from build123d import *

# Parameters (mm, degrees)
PAD004_DEPTH = 0.25
PAD003_DEPTH = 0.25
PAD005_DEPTH = 0.25
PAD008_DEPTH = 0.3
SKETCH008_W  = 4.5
SKETCH008_H  = 0.35
PAD006_DEPTH = 4
PAD001_DEPTH = 0.18
PAD002_DEPTH = 0.25
PAD007_DEPTH = 0.3
SKETCH_W     = 10
SKETCH_H     = 6.5
PAD_DEPTH    = 4.7
POCKET_DEPTH = 0.5
FILLET_R     = 0.2


with BuildPart() as pad004:
    # Sketch006 → Pad004 (new body, symmetric)
    with BuildSketch(Plane.XZ.offset(-3.8)):
        with BuildLine():
            Line((-3.9, 0), (-3.549998, 0))
            ThreePointArc((-3.549998, 0), (-3.196446, 0.146447), (-3.05, 0.5))
            Line((-3.05, 1.6), (-3.05, 0.5))
            Line((-3.3, 1.6), (-3.05, 1.6))
            Line((-3.3, 0.499998), (-3.3, 1.6))
            ThreePointArc((-3.549998, 0.25), (-3.373223, 0.323223), (-3.3, 0.499998))
            Line((-3.549998, 0.25), (-3.9, 0.25))
            Line((-3.9, 0.25), (-3.9, 0))
        make_face()
        with BuildLine():
            Line((3.3, 1.6), (3.05, 1.6))
            Line((3.05, 1.6), (3.05, 0.500004))
            ThreePointArc((3.05, 0.500004), (3.196444, 0.146448), (3.549998, 0))
            Line((3.9, 0), (3.549998, 0))
            Line((3.9, 0.25), (3.9, 0))
            Line((3.549998, 0.25), (3.9, 0.25))
            ThreePointArc((3.3, 0.499998), (3.373223, 0.323223), (3.549998, 0.25))
            Line((3.3, 0.499998), (3.3, 1.6))
        make_face()
    extrude(amount=PAD004_DEPTH, both=True)


with BuildPart() as pad003:
    # Sketch005 → Pad003 (new body, symmetric)
    with BuildSketch(Plane.XZ.offset(3.8)):
        with BuildLine():
            Line((-3.9, 0), (-3.549998, 0))
            ThreePointArc((-3.549998, 0), (-3.196446, 0.146447), (-3.05, 0.5))
            Line((-3.05, 1.6), (-3.05, 0.5))
            Line((-3.3, 1.6), (-3.05, 1.6))
            Line((-3.3, 0.499998), (-3.3, 1.6))
            ThreePointArc((-3.549998, 0.25), (-3.373223, 0.323223), (-3.3, 0.499998))
            Line((-3.549998, 0.25), (-3.9, 0.25))
            Line((-3.9, 0.25), (-3.9, 0))
        make_face()
        with BuildLine():
            Line((3.3, 1.6), (3.05, 1.6))
            Line((3.05, 1.6), (3.05, 0.500004))
            ThreePointArc((3.05, 0.500004), (3.196444, 0.146448), (3.549998, 0))
            Line((3.9, 0), (3.549998, 0))
            Line((3.9, 0.25), (3.9, 0))
            Line((3.549998, 0.25), (3.9, 0.25))
            ThreePointArc((3.3, 0.499998), (3.373223, 0.323223), (3.549998, 0.25))
            Line((3.3, 0.499998), (3.3, 1.6))
        make_face()
    extrude(amount=PAD003_DEPTH, both=True)


with BuildPart() as pad005:
    # Sketch007 → Pad005 (new body, symmetric)
    with BuildSketch(Plane.XZ.offset(-0.61)):
        with BuildLine():
            Line((-3.9, 0), (-3.549998, 0))
            ThreePointArc((-3.549998, 0), (-3.196446, 0.146447), (-3.05, 0.5))
            Line((-3.05, 1.6), (-3.05, 0.5))
            Line((-3.3, 1.6), (-3.05, 1.6))
            Line((-3.3, 0.499998), (-3.3, 1.6))
            ThreePointArc((-3.549998, 0.25), (-3.373223, 0.323223), (-3.3, 0.499998))
            Line((-3.549998, 0.25), (-3.9, 0.25))
            Line((-3.9, 0.25), (-3.9, 0))
        make_face()
        with BuildLine():
            Line((3.3, 1.6), (3.05, 1.6))
            Line((3.05, 1.6), (3.05, 0.500004))
            ThreePointArc((3.05, 0.500004), (3.196444, 0.146448), (3.549998, 0))
            Line((3.9, 0), (3.549998, 0))
            Line((3.9, 0.25), (3.9, 0))
            Line((3.549998, 0.25), (3.9, 0.25))
            ThreePointArc((3.3, 0.499998), (3.373223, 0.323223), (3.549998, 0.25))
            Line((3.3, 0.499998), (3.3, 1.6))
        make_face()
    extrude(amount=PAD005_DEPTH, both=True)


with BuildPart() as pad008:
    # Sketch010 → Pad008 (new body)
    with BuildSketch(Plane.XZ.offset(-5)):
        Polygon((-1.75, 0.3), (1.75, 0.3), (2.25, 0.85), (-2.25, 0.85), align=None)
    extrude(amount=PAD008_DEPTH)


with BuildPart() as pad006:
    # Sketch008 → Pad006 (new body, symmetric)
    with BuildSketch(Plane.XZ):
        with Locations((0, 0.675)):
            Rectangle(SKETCH008_W, SKETCH008_H)
    extrude(amount=PAD006_DEPTH, both=True)


with BuildPart() as pad001:
    # Sketch001 → Pad001 (new body)
    with BuildSketch(Plane(origin=(0, 0, 5.4), x_dir=(0, -1, 0), z_dir=(0, 0, 1))):
        with BuildLine():
            Line((-3.8, -1.8), (-3.8, 2.2))
            ThreePointArc((-3.8, 2.2), (-4, 2.4), (-4.2, 2.2))
            Line((-4.2, 2.2), (-4.2, -1.8))
            ThreePointArc((-4.2, -1.8), (-4, -2), (-3.8, -1.8))
        make_face()
    extrude(amount=PAD001_DEPTH)


with BuildPart() as pad002:
    # Sketch004 → Pad002 (new body, symmetric)
    with BuildSketch(Plane.XZ.offset(1.59)):
        with BuildLine():
            Line((-3.9, 0), (-3.549998, 0))
            ThreePointArc((-3.549998, 0), (-3.196446, 0.146447), (-3.05, 0.5))
            Line((-3.05, 1.6), (-3.05, 0.5))
            Line((-3.3, 1.6), (-3.05, 1.6))
            Line((-3.3, 0.499998), (-3.3, 1.6))
            ThreePointArc((-3.549998, 0.25), (-3.373223, 0.323223), (-3.3, 0.499998))
            Line((-3.549998, 0.25), (-3.9, 0.25))
            Line((-3.9, 0.25), (-3.9, 0))
        make_face()
        with BuildLine():
            Line((3.3, 1.6), (3.05, 1.6))
            Line((3.05, 1.6), (3.05, 0.500004))
            ThreePointArc((3.05, 0.500004), (3.196444, 0.146448), (3.549998, 0))
            Line((3.9, 0), (3.549998, 0))
            Line((3.9, 0.25), (3.9, 0))
            Line((3.549998, 0.25), (3.9, 0.25))
            ThreePointArc((3.3, 0.499998), (3.373223, 0.323223), (3.549998, 0.25))
            Line((3.3, 0.499998), (3.3, 1.6))
        make_face()
    extrude(amount=PAD002_DEPTH, both=True)


with BuildPart() as pad007:
    # Sketch009 → Pad007 (new body)
    with BuildSketch(Plane.XZ.offset(5)):
        Polygon((-1.75, 0.3), (1.75, 0.3), (2.25, 0.85), (-2.25, 0.85), align=None)
    extrude(amount=-PAD007_DEPTH)


with BuildPart() as obj1:
    # Sketch → Pad (new body)
    with BuildSketch(Plane(origin=(0, 0, 0.8), x_dir=(0, -1, 0), z_dir=(0, 0, 1))):
        Rectangle(SKETCH_W, SKETCH_H)
    extrude(amount=PAD_DEPTH)

    # Sketch003 → Pocket (cut)
    with BuildSketch(Plane(origin=(0, 0, 5.5), x_dir=(0, -1, 0), z_dir=(0, 0, 1))):
        with BuildLine():
            ThreePointArc((-0.318267, 7.6), (0.223846, 7.813173), (0.45, 8.35))
            Line((0.45, 8.35), (-2.05, 8.35))
            Line((-2.05, 8.35), (-2.05, 7.6))
            Line((-2.05, 7.6), (-0.318267, 7.6))
        make_face()
        with BuildLine():
            Line((9.6, -0.75), (12.1, -0.75))
            Line((12.1, -0.75), (12.1, 0))
            Line((10.285847, 0), (12.1, 0))
            ThreePointArc((10.285847, 0), (9.797313, -0.241845), (9.6, -0.75))
        make_face()
    extrude(amount=-POCKET_DEPTH, mode=Mode.SUBTRACT)

    # Fillet
    fillet_edges = [obj1.edges().sort_by_distance(p)[0] for p in [
        (-3.25, 0, 5.5),
        (0, -5, 5.5),
        (3.25, 0, 5.5),
        (0, 5, 5.5),
    ]]
    fillet(fillet_edges, radius=FILLET_R)

    add(pad004.part)
    add(pad003.part)
    add(pad005.part)
    add(pad008.part)
    add(pad006.part)
    add(pad001.part)
    add(pad002.part)
    add(pad007.part)


solid = obj1.part
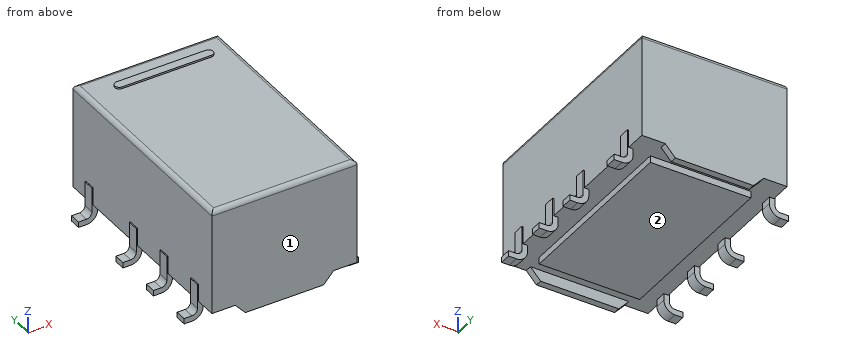
Design review of the part built by this model. Coordinates are the model's own, in mm. Face numbers are marked on the shaded views. Give positions to 0.01 mm unless a question says otherwise; leave off trailing zeros. Write each loop counter-clockwise with the first axis right and the second up, starting at its lowest first coordinate (ties: lowest second). Pieces come first, ordered by that corner, then holes. Notation, with made-up numbers: M 30.25,-7 L 76.25,-7 A20 ccw 76.25,19 Z; hole C -31.75,47 d8. An arc over 180 degrees is marked long. Answer as a JSON object with one key per item and string values. Group by question number.
1) We need section C-C (z = 3.1). Give the boundary of the cut face in (x, y).
2) For line 1 along Z through (x, y) = (-2.5, -4); line 2 along X through (y, z) = (4.5, 2.5); line 3 along Z through (x, y) = (1.75, -1.5), list the stretches that pass through material, from the lowest coordinate up.
3) We need section B-B (x = -0.75). Give the boundary of the cut face in (y, z).
4) We need section D-D (x = 2.75). Give the boundary of the cut face in (y, z).
5) Clearance check with flat-ended pins moving along their axes: pin 1 Ø1 at (y, z) = (1, 4) entering from +X; pin 2 Ø2 at (x, y) = (1, 0) entering from -Z. State where each tip first meets the part, or that it passes through.
6) We need section A-A (y = -2.25). Give the boundary of the cut face in (x, z), and give its area (3 significant figures).
7) Mouldability with a two-part tool opening along X and no side actions: class the marked faces 1 and 2 as released by +X, released by -X, zero draft, split by the parting line, or undercut.
Answer key:
{
 "1": {"outline": "M -3.25,-5 L 3.25,-5 L 3.25,5 L -3.25,5 Z"},
 "2": {"line 1": "z = 0.8 to 5.5", "line 2": "x = -3.25 to 3.25", "line 3": "z = 0.5 to 5.5"},
 "3": {"outline": "M -5,0.3 L -4.7,0.3 L -4.7,0.8 L -4,0.8 L -4,0.5 L 4,0.5 L 4,0.8 L 4.7,0.8 L 4.7,0.3 L 5,0.3 L 5,5.3 A0.2 ccw 4.8,5.5 L 4.2,5.5 L 4.2,5.58 L 3.8,5.58 L 3.8,5.5 L -4.8,5.5 A0.2 ccw -5,5.3 Z"},
 "4": {"outline": "M -5,0.8 L 5,0.8 L 5,5.3 A0.2 ccw 4.8,5.5 L -4.8,5.5 A0.2 ccw -5,5.3 Z"},
 "5": {"pin 1": "stops at x = 3.25", "pin 2": "stops at z = 0.5"},
 "6": {"outline": "M -3.25,0.8 L -2.25,0.8 L -2.25,0.5 L 2.25,0.5 L 2.25,0.8 L 3.25,0.8 L 3.25,5.3 A0.2 ccw 3.05,5.5 L -3.05,5.5 A0.2 ccw -3.25,5.3 Z", "area": "31.9 mm²"},
 "7": {"face 1": "zero draft", "face 2": "undercut"}
}
